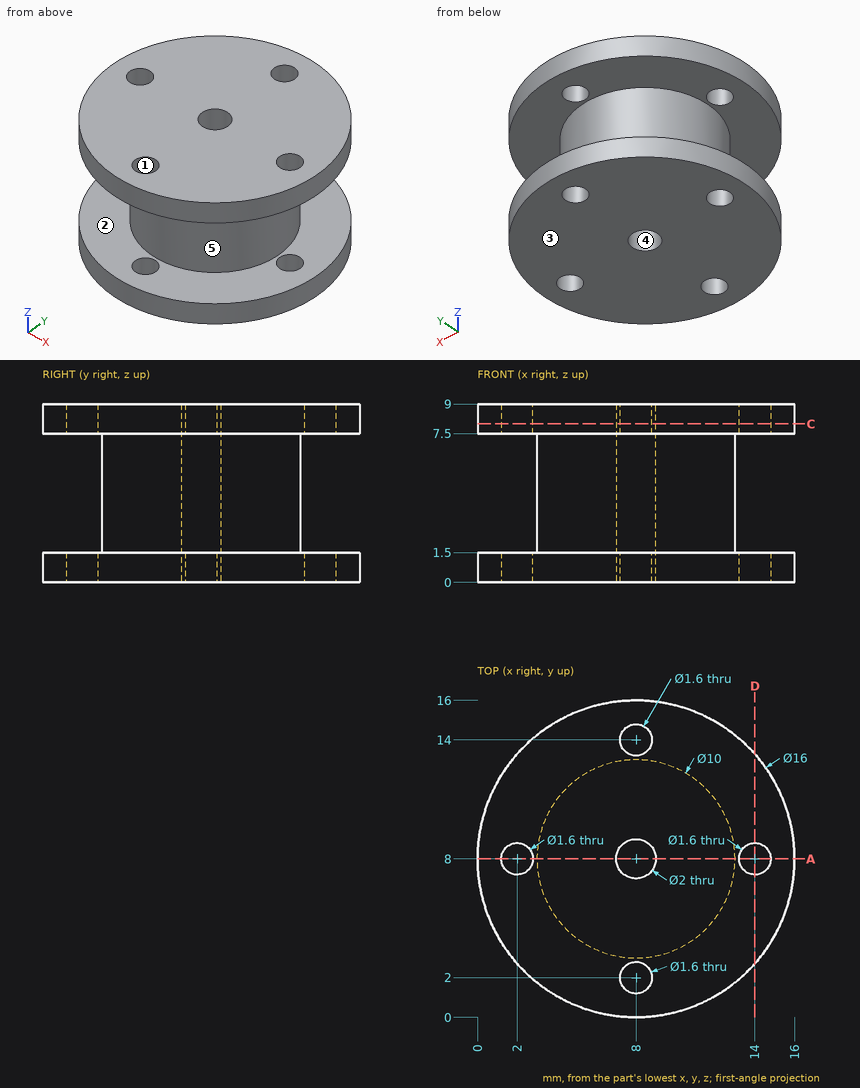
The drawing under review shows one solid part. Ordinate dimensions are in mm from its lowest x, y, z. A direction names the side the tool comes from. Coordinates: 2 decimals unless noted, no trailing zeros. Loops run counter-clockwise (first coordinate to the right, second up) from the corner with the lowest first, then second, coordinate; pieces in that order, holes last. Notation, with made-up numbers: M 21,-20 L 31,-20 A20 ccw 31,8 Z; hole C 31.5,76.25 d5. An arc over 180 degrees is marked long. Use one line per item in the form item = value.
(1) Draft analysis for pull direction Y (two halves, no side actions). For the marked faces 3, 4 and 5, state which applies: pulls with the +Y half, pulls with the -Y half, needs draft (parallel to the pull), parting line crosses it, or undercut.
Return value:
face_3 = needs draft
face_4 = undercut
face_5 = parting line crosses it
(2) Consider section D-D (x = 14). Write out the cut boundary in (y, z).
Return value:
outline = M 2.71,0 L 7.2,0 L 7.2,1.5 L 2.71,1.5 Z; M 2.71,7.5 L 7.2,7.5 L 7.2,9 L 2.71,9 Z; M 8.8,0 L 13.29,0 L 13.29,1.5 L 8.8,1.5 Z; M 8.8,7.5 L 13.29,7.5 L 13.29,9 L 8.8,9 Z
(3) For the marked faces 1 and 2, list the 3-axis set-ups (+Z, -Z, +X, -X, +Y, -Y) from which the entire face can be reached by the end or side of a thin tool; tool diameter is ignored.
Return value:
face_1 = +Z, -Z
face_2 = none
(4) For line 1 along Y through (x, z) = (8, 8.6); line 2 along Z through (x, y) = (14.5, 12); line 3 along Y through (x, z) = (8, 3.75), list the stretches that pass through material, from the lowest coordinate up. Write a range as from..to.
Return value:
line_1 = 0..1.2, 2.8..7, 9..13.2, 14.8..16
line_2 = 0..1.5, 7.5..9
line_3 = 3..7, 9..13
(5) Consider section C-C (z = 8). Write out the cut boundary in (x, y).
Return value:
outline = C 8,8 d16; hole C 2,8 d1.6; hole C 8,8 d2; hole C 8,2 d1.6; hole C 8,14 d1.6; hole C 14,8 d1.6
(6) Clearance check with flat-ended pins moving along their axes: P1, Ø3, axis at y = 14, z = 5, coming from the +X side; P2, Ø3, axis at y = 5, z = 6.5, coming from the -X side. State where each tip first meets the part, or that it passes through.
Return value:
P1 = 10.18
P2 = 0.22
(7) Consider section A-A (y = 8). Give the number of separate pieces and of enclosed holes in the cut face, and give its area (3 significant figures).
Return value:
separate_pieces = 6
enclosed_holes = 0
area = 80.4 mm2
